Build history of the part. All positions in model axes, mm. Face numbers are marked on the shaded views. A direction names the side the tool comes from. Give positions to 0.01 mm unless a question says otherwise; leave off trailing zeros. Order: outer loops, then holes, each group sorted by start corner. A loop starts at its lowest first (then second) coordinate and runs counter-clockwise, first axis right, second up. Notation, with made-up numbers: (-17, 82.25) - (37, 82.25) arc R12 cw to (37, 89.25) - close; hole circle Ø7 at (25, 21). An arc over 180 degrees is marked (long way). Use a Markdown table: item, result.
from build123d import *

# Parameters (mm, degrees)
PAD_DEPTH       = 3
SKETCH001_R     = 9
PAD001_DEPTH    = 10
SKETCH002_R     = 8.2
PAD002_DEPTH    = 1.3
SKETCH003_R     = 1
PAD003_DEPTH    = 2.5
SKETCH004_R     = 1
POCKET_DEPTH    = 3
SKETCH005_R     = 1
POCKET001_DEPTH = 3
SKETCH006_R     = 2
PAD004_DEPTH    = 0.6
SKETCH007_R     = 1
PAD005_DEPTH    = 1
SKETCH008_W     = 5
SKETCH008_H     = 2
PAD006_DEPTH    = 8


with BuildPart() as part:
    # Sketch → Pad (new body)
    with BuildSketch(Plane.XY):
        with BuildLine():
            ThreePointArc((3.450971, -4.263113), (6.482051, -3.742414), (5.41745, -0.857073))
            Line((5.41745, -0.857073), (3.748487, 0.106503))
            ThreePointArc((3.748487, 0.106503), (3.247595, 1.875), (1.966478, 3.193034))
            Line((1.966478, 5.120185), (1.966478, 3.193034))
            ThreePointArc((1.966478, 5.120185), (0, 7.484828), (-1.966478, 5.120185))
            Line((-1.966478, 5.120185), (-1.966478, 3.193034))
            ThreePointArc((-1.966478, 3.193034), (-3.247595, 1.875), (-3.748487, 0.106503))
            Line((-5.41745, -0.857073), (-3.748487, 0.106503))
            ThreePointArc((-5.41745, -0.857073), (-6.482051, -3.742414), (-3.450971, -4.263113))
            Line((-3.450971, -4.263113), (-1.782009, -3.299537))
            ThreePointArc((-1.782009, -3.299537), (0, -3.75), (1.782009, -3.299537))
            Line((3.450971, -4.263113), (1.782009, -3.299537))
        make_face()
    extrude(amount=PAD_DEPTH)

    # Sketch001 (on Face14 of Pad) → Pad001 (join)
    with BuildSketch(Plane.XY.offset(3)):
        Circle(SKETCH001_R)
    extrude(amount=PAD001_DEPTH)

    # Sketch002 (on Face3 of Pad001) → Pad002 (join)
    with BuildSketch(Plane.XY.offset(13)):
        Circle(SKETCH002_R)
    extrude(amount=PAD002_DEPTH)

    # Sketch003 (on Face18 of Pad002) → Pad003 (join)
    with BuildSketch(Plane.XY.offset(14.3)):
        Circle(SKETCH003_R)
    extrude(amount=PAD003_DEPTH)

    # Sketch004 (on Face17 of Pad003) → Pocket (cut)
    with BuildSketch(Plane(origin=(0, 0, 0), x_dir=(1, 0, 0), z_dir=(0, 0, -1))):
        with Locations((4.75, 2.742414)):
            Circle(SKETCH004_R)
        with Locations((-4.75, 2.742414)):
            Circle(SKETCH004_R)
        with Locations((0, -5.484828)):
            Circle(SKETCH004_R)
    extrude(amount=-POCKET_DEPTH, mode=Mode.SUBTRACT)

    # Sketch005 (on Face18 of Pocket) → Pocket001 (cut)
    with BuildSketch(Plane.XY.offset(14.3)):
        with Locations((0, 5.5)):
            Circle(SKETCH005_R)
        with Locations((0, -5.5)):
            Circle(SKETCH005_R)
        with BuildLine():
            ThreePointArc((-2.12132, 2.12132), (-3, 0), (-2.12132, -2.12132))
            ThreePointArc((-4.949764, -4.949731), (-2.121328, -4.949756), (-2.12132, -2.12132))
            ThreePointArc((-4.949748, 4.949747), (-7, 1.1e-05), (-4.949764, -4.949731))
            ThreePointArc((-2.12132, 2.12132), (-2.12132, 4.949747), (-4.949748, 4.949747))
        make_face()
        with BuildLine():
            ThreePointArc((2.12132, -2.12132), (3, 0), (2.12132, 2.12132))
            ThreePointArc((4.949748, 4.949747), (2.12132, 4.949748), (2.12132, 2.12132))
            ThreePointArc((4.949747, -4.949748), (7, 0), (4.949748, 4.949747))
            ThreePointArc((2.12132, -2.12132), (2.12132, -4.949747), (4.949747, -4.949748))
        make_face()
    extrude(amount=-POCKET001_DEPTH, mode=Mode.SUBTRACT)

    # Sketch006 (on Face17 of Pocket001) → Pad004 (join)
    with BuildSketch(Plane(origin=(0, 0, 0), x_dir=(1, 0, 0), z_dir=(0, 0, -1))):
        Circle(SKETCH006_R)
    extrude(amount=PAD004_DEPTH)

    # Sketch007 (on Face36 of Pad004) → Pad005 (join)
    with BuildSketch(Plane(origin=(0, 0, -0.6), x_dir=(1, 0, 0), z_dir=(0, 0, -1))):
        Circle(SKETCH007_R)
    extrude(amount=PAD005_DEPTH)

    # Sketch008 (on Face2 of Pad005) → Pad006 (join)
    with BuildSketch(Plane(origin=(0, 0, 3), x_dir=(1, 0, 0), z_dir=(0, 0, -1))):
        with Locations((0, 4.75)):
            Rectangle(SKETCH008_W, SKETCH008_H)
    extrude(amount=PAD006_DEPTH)


solid = part.part
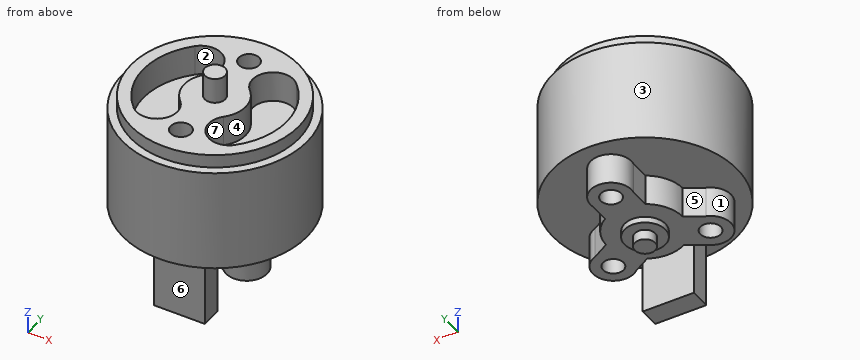
1) Wall check: line 1 (Y direction, x = 0, z = 13.3); line 2 (Y direction, x = 0, z = 12.2); line 3 (X direction, y = -1.5, z = 14). Give the ranges that are in metal, low to high. Write a range as from..to.
Computed:
| item | result |
|---|---|
| line 1 | y = -8.2..-6.5, -4.5..4.5, 6.5..8.2 |
| line 2 | y = -9..-6.5, -4.5..4.5, 6.5..9 |
| line 3 | x = -8.06..-6.84, -2.6..2.6, 6.84..8.06 |
2) Two-plate mould, pull along Y, no slides. Class the marked faces 4, 5, 6 and 7: +Y half, -Y half, draft (parallel to the pull), parting line (faces both ways), or undercut.
Computed:
| item | result |
|---|---|
| face 4 | undercut |
| face 5 | +Y half |
| face 6 | -Y half |
| face 7 | undercut |
3) Slice it at A-A (y = 2.5). Write the cut outline in (x, z).
Computed:
| item | result |
|---|---|
| outline | (-8.65, 3) - (-2.8, 3) - (-2.8, 0) - (2.8, 0) - (2.8, 3) - (8.65, 3) - (8.65, 13) - (7.81, 13) - (7.81, 14.3) - (6.54, 14.3) - (6.54, 11.3) - (1.82, 11.3) - (1.82, 14.3) - (-1.82, 14.3) - (-1.82, 11.3) - (-6.54, 11.3) - (-6.54, 14.3) - (-7.81, 14.3) - (-7.81, 13) - (-8.65, 13) - close |
4) Tool access for the marked faces 1, 2 and 3: list every direction of +Z, -Z, +X, -X, +Y, -Y with a clear straight run to the whole face (end or side of a thin tool).
Computed:
| item | result |
|---|---|
| face 1 | -Z |
| face 2 | +Z |
| face 3 | +Z, -Z |
5) Pin check, flat tips, straight feed: P1, Ø8, axis at x = -5.5, z = 13, coming from the +Y side; P2, Ø4, axis at x = -1, z = 0, coming from the +Y side; P3, Ø1.6, axis at y = -4.5, z = 0, coming from the +X side. Stop position of each tip, or through.
Computed:
| item | result |
|---|---|
| P1 | stops at y = 8.87 |
| P2 | stops at y = 7.48 |
| P3 | stops at x = 6.51 |
6) Slice it at B-B (z = 8). Write the cut outline in (x, y).
Computed:
| item | result |
|---|---|
| outline | circle Ø18 at (0, 0) |
7) Slice it at C-C (z = 15.5). Write the cut outline in (x, y).
Computed:
| item | result |
|---|---|
| outline | circle Ø2 at (0, 0) |
8) Slice it at D-D (z = -3.25). Write the cut outline in (x, y), and give its area (3 significant figures).
Computed:
| item | result |
|---|---|
| outline | (-2.5, -5.75) - (2.5, -5.75) - (2.5, -3.75) - (-2.5, -3.75) - close |
| area | 10.0 mm² |
